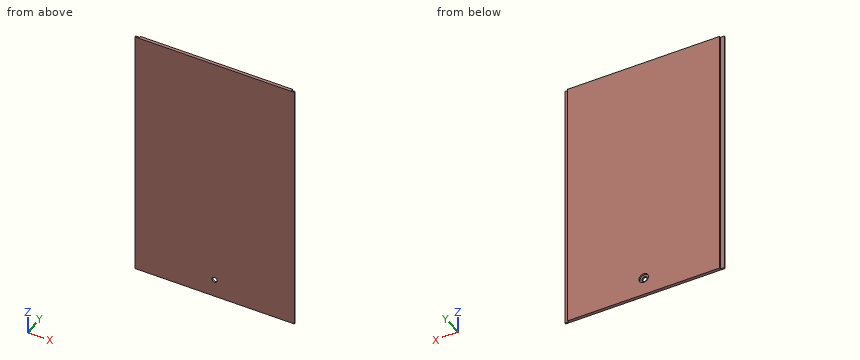
```python
from build123d import *

# Parameters (mm, degrees)
SKETCH_1_W          = 76.15
SKETCH_1_H          = 127.3
EXTRUDE_1_DEPTH     = 1.5
SKETCH_2_W          = 1.9
SKETCH_2_H          = 0.7
EXTRUDE_2_DEPTH     = 127.3
SKETCH_3_R          = 1.3
CUT_EXTRUDE_1_DEPTH = 76.176945435
SKETCH_5_R          = 2.375
CUT_EXTRUDE_2_DEPTH = 0.8


with BuildPart() as part:
    # Эскиз1 → Бобышка-Вытянуть1 (new body)
    with BuildSketch(Plane(origin=(0, 0, 0), x_dir=(1, 0, 0), z_dir=(0, 1, 0))):
        Rectangle(SKETCH_1_W, SKETCH_1_H)
    extrude(amount=EXTRUDE_1_DEPTH)

    # Эскиз2 → Бобышка-Вытянуть2 (add)
    with BuildSketch(Plane.XY.offset(63.65)):
        with Locations((-39.025, 0.35)):
            Rectangle(SKETCH_2_W, SKETCH_2_H)
        with Locations((39.025, 0.35)):
            Rectangle(SKETCH_2_W, SKETCH_2_H)
    extrude(amount=-EXTRUDE_2_DEPTH)

    # Эскиз3 → Вырез-Вытянуть1 (cut, through all)
    with BuildSketch(Plane(origin=(0, 1.5, 0), x_dir=(1, 0, 0), z_dir=(0, 1, 0))):
        with Locations(Location((0, 54.65, 0), (0, 0, 270))):
            Circle(SKETCH_3_R)
    extrude(amount=-CUT_EXTRUDE_1_DEPTH, mode=Mode.SUBTRACT)

    # Эскиз5 → Вырез-Вытянуть2 (cut)
    with BuildSketch(Plane(origin=(0, 1.5, 0), x_dir=(1, 0, 0), z_dir=(0, 1, 0))):
        with Locations(Location((0, 54.65, 0), (0, 0, 270))):
            Circle(SKETCH_5_R)
    extrude(amount=-CUT_EXTRUDE_2_DEPTH, mode=Mode.SUBTRACT)


solid = part.part
```
Geometry check sheet. Reference: the model listing, model coordinates, mm. Coordinates: 2 decimals unless noted, no trailing zeros. Write each loop counter-clockwise with the first axis right and the second up, starting at its lowest first coordinate (ties: lowest second). Pieces come first, ordered by that corner, then holes. Notation, with made-up numbers: M 79,22.25 L 90,22.25 A9 ccw 90,32.25 Z; hole C 84.5,52 d11. An arc over 180 degrees is marked long. Use one line per item in the form item = value. Start each with the question number.
1) Section check B-B on x = 0. Enter the section's corners in (y, z) (3 decimals), and give its area (3 significant figures).
2) Go/stop test with flat-tipped pins: pin 1 Ø2 at (x, z) = (38.5, 14.5) entering from +Y; pin 2 Ø1 at (x, z) = (-39, 22.5) entering from +Y. Record where each tip stops, or that it passes through.
3) Thickness scan on probe 1 along X at (y, z) = (0.55, -54.65) (3 decimals); probe 2 along X at (y, z) = (1.1, -54.65) (3 decimals); probe 3 along X at (y, z) = (1.2, 40) (3 decimals). Record the ranges inside material, lowest first. Write a range as from..to.
4) Section check A-A on z = -54.65. Enter the section's corners in (x, y) (3 decimals).
5) Section check C-C on z = -24. Enter the section's corners in (x, y) (3 decimals), and give its area (3 significant figures).
Responses:
q1.outline = M 0,-63.65 L 1.5,-63.65 L 1.5,-57.025 L 0.7,-57.025 L 0.7,-55.95 L 0,-55.95 Z; M 0,-53.35 L 0.7,-53.35 L 0.7,-52.275 L 1.5,-52.275 L 1.5,63.65 L 0,63.65 Z
q1.area = 185 mm2
q2.pin_1 = 1.5
q2.pin_2 = 0.7
q3.probe_1 = -39.975..-1.3, 1.3..39.975
q3.probe_2 = -38.075..-2.375, 2.375..38.075
q3.probe_3 = -38.075..38.075
q4.outline = M -39.975,0 L -1.3,0 L -1.3,0.7 L -2.375,0.7 L -2.375,1.5 L -38.075,1.5 L -38.075,0.7 L -39.975,0.7 Z; M 1.3,0 L 39.975,0 L 39.975,0.7 L 38.075,0.7 L 38.075,1.5 L 2.375,1.5 L 2.375,0.7 L 1.3,0.7 Z
q5.outline = M -39.975,0 L 39.975,0 L 39.975,0.7 L 38.075,0.7 L 38.075,1.5 L -38.075,1.5 L -38.075,0.7 L -39.975,0.7 Z
q5.area = 117 mm2
